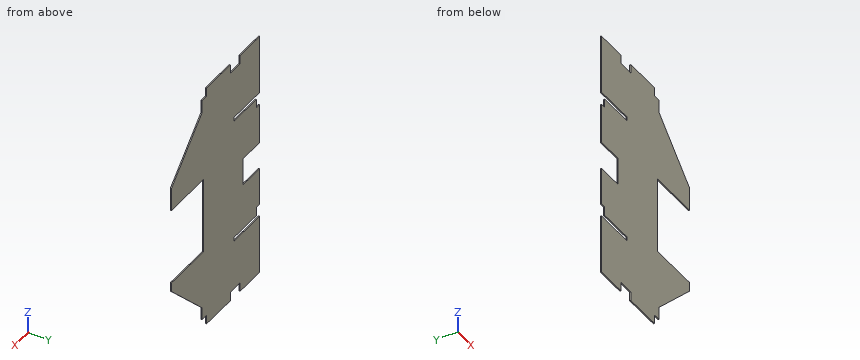
Autodesk Inventor part; units mm, degrees
ref_plane "YZ Plane" through (0, 0, 0) normal (1, 0, 0) x (0, 1, 0)
ref_plane "XZ Plane" through (0, 0, 0) normal (0, 1, 0) x (-1, 0, 0)
ref_plane "XY Plane" through (0, 0, 0) normal (0, 0, 1) x (1, 0, 0)
sketch "Sketch1" plane through (0, 0, 0) normal (0, 1, 0) x (-1, 0, 0)
  line L0 (234.95, 355.6) -> (-234.95, 355.6)
  line L1 (-234.95, 355.6) -> (-234.95, -355.6)
  line L2 (-234.95, -355.6) -> (234.95, -355.6)
  line L3 (234.95, -355.6) -> (234.95, 355.6)
  line L4 (234.95, 355.6) -> (-234.95, -355.6) construction
  line L5 (-234.95, 355.6) -> (234.95, -355.6) construction
  point P0 (0, 0)
  dimension "d0" = 469.9
  dimension "d1" = 711.2
extrude "Plate1" add sketch "Sketch1" along normal blind 3.048
sketch "Sketch3" plane through (0, 3.048, 0) normal (0, 1, 0) x (1, 0, 0)
  line L0 (234.95, -355.6) -> (-234.95, -355.6)
  point P0 (0, 0)
sketch "Sketch4" plane through (0, 0, 0) normal (0, -1, 0) x (1, 0, 0)
  line L0 (-234.95, 355.6) -> (234.95, 355.6)
  line L1 (-234.95, -355.6) -> (-234.95, 355.6)
  line L2 (234.95, -355.6) -> (-234.95, -355.6)
  line L3 (234.95, 355.6) -> (234.95, -355.6)
  line L4 (-234.95, 355.6) -> (234.95, 355.6)
  line L5 (25.4, 355.6) -> (25.4, 294.64)
  line L6 (165.1, 101.6) -> (234.95, 101.6)
  line L7 (234.95, 355.6) -> (234.95, -355.6)
  line L8 (25.4, 294.64) -> (165.1, 154.94)
  line L9 (25.4, 294.64) -> (222.9656, 294.64) construction
  line L10 (165.1, 154.94) -> (165.1, 101.6)
  line L11 (234.95, 0) -> (-234.95, 0)
  line L12 (-234.95, -355.6) -> (-234.95, 355.6)
  line L13 (25.4, -355.6) -> (25.4, -294.64)
  line L14 (165.1, -127) -> (234.95, -127)
  line L15 (25.4, -294.64) -> (165.1, -154.94)
  line L16 (25.4, -294.64) -> (222.9656, -294.64) construction
  line L17 (165.1, -154.94) -> (165.1, -127)
  line L18 (-234.95, 184.15) -> (-120.65, 184.15)
  line L19 (-120.65, 184.15) -> (-120.65, 177.8)
  line L20 (-120.65, 177.8) -> (-222.25, 177.8)
  line L21 (-222.25, 177.8) -> (-222.25, 152.4)
  line L22 (-222.25, 152.4) -> (-234.95, 152.4)
  line L23 (-234.95, 149.86) -> (-219.71, 149.86)
  line L24 (-219.71, 149.86) -> (-219.71, 175.26)
  line L25 (-219.71, 175.26) -> (-118.11, 175.26)
  line L26 (-118.11, 175.26) -> (-118.11, 186.69)
  line L27 (-118.11, 186.69) -> (-234.95, 186.69)
  line L28 (165.1, -129.54) -> (20.32, -129.54)
  line L29 (20.32, -129.54) -> (20.32, 88.9)
  line L30 (20.32, 88.9) -> (165.1, 88.9)
  line L31 (165.1, 101.6) -> (165.1, 88.9)
  line L32 (-234.95, -184.15) -> (-120.65, -184.15)
  line L33 (-120.65, -184.15) -> (-120.65, -177.8)
  line L34 (-120.65, -177.8) -> (-222.25, -177.8)
  line L35 (-222.25, -177.8) -> (-222.25, -152.4)
  line L36 (-222.25, -152.4) -> (-234.95, -152.4)
  line L37 (-234.95, -149.86) -> (-219.71, -149.86)
  line L38 (-219.71, -149.86) -> (-219.71, -175.26)
  line L39 (-219.71, -175.26) -> (-118.11, -175.26)
  line L40 (-118.11, -175.26) -> (-118.11, -186.69)
  line L41 (-118.11, -186.69) -> (-234.95, -186.69)
  line L42 (-158.75, 35.56) -> (-158.75, -43.18)
  line L43 (-158.75, -43.18) -> (-234.95, -43.18)
  line L44 (-158.75, 35.56) -> (-234.95, 35.56)
  line L45 (25.4, 330.2) -> (6.35, 330.2)
  line L46 (6.35, 330.2) -> (6.35, 355.6)
  line L47 (25.4, -330.2) -> (6.35, -330.2)
  line L48 (6.35, -330.2) -> (6.35, -355.6)
  line L49 (234.95, -355.6) -> (-234.95, -355.6)
  point P0 (0, 0)
  dimension "d3" = 209.55
  dimension "d4" = 254
  dimension "d5" = 45
  dimension "d6" = 60.96
  dimension "d9" = 69.85
  dimension "d12" = 45
  dimension "d13" = 209.55
  dimension "d14" = 228.6
  dimension "d15" = 69.85
  dimension "d16" = 60.96
  dimension "d17" = 171.45
  dimension "d18" = 114.3
  dimension "d19" = 6.35
  dimension "d21" = 101.6
  dimension "d22" = 25.4
  dimension "d23" = 2.54
  dimension "d26" = 144.78
  dimension "d31" = 12.7
  dimension "d32" = 114.3
  dimension "d33" = 171.45
  dimension "d34" = 6.35
  dimension "d35" = 101.6
  dimension "d36" = 25.4
  dimension "d37" = 2.54
  dimension "d38" = 76.2
  dimension "d39" = 35.56
  dimension "d40" = 43.18
  dimension "d41" = 2.54
  dimension "d42" = 25.4
  dimension "d43" = 19.05
  dimension "d44" = 25.4
  dimension "d45" = 19.05
extrude "Cut1" cut sketch "Sketch4" against normal blind 3.048 contours L27 L26 L25 L24 L23 L1 L22 L21 L20 L19 L18 | L0 L3 L6 L10 L8 L5 | L18 L19 L20 L21 L22 L1 | L3 L11 L29 L30 L31 L6 | L3 L14 L17 L28 L29 L11 | L44 L42 L11 L1 | L3 L2 L13 L15 L17 L14 | L11 L42 L43 L1 | L37 L38 L39 L40 L41 L1 L32 L33 L34 L35 L36 | L36 L35 L34 L33 L32 L1
sketch "Sketch5" plane through (0, 0, 0) normal (0, -1, 0) x (1, 0, 0)
  line L0 (25.4, 355.6) -> (25.4, 294.64)
  line L1 (25.4, 294.64) -> (165.1, 154.94)
  line L2 (165.1, 154.94) -> (165.1, 88.9)
  line L3 (165.1, 88.9) -> (20.32, 88.9)
  line L4 (20.32, 88.9) -> (20.32, -129.54)
  line L5 (20.32, -129.54) -> (165.1, -129.54)
  line L6 (165.1, -129.54) -> (165.1, -154.94)
  line L7 (165.1, -154.94) -> (25.4, -294.64)
  line L8 (25.4, -294.64) -> (25.4, -355.6)
  line L9 (25.4, -355.6) -> (-234.95, -355.6)
  line L10 (-234.95, -355.6) -> (-234.95, -186.69)
  line L11 (-234.95, -186.69) -> (-118.11, -186.69)
  line L12 (-118.11, -186.69) -> (-118.11, -175.26)
  line L13 (-118.11, -175.26) -> (-219.71, -175.26)
  line L14 (-219.71, -175.26) -> (-219.71, -149.86)
  line L15 (-219.71, -149.86) -> (-234.95, -149.86)
  line L16 (-234.95, -149.86) -> (-234.95, -43.18)
  line L17 (-234.95, -43.18) -> (-158.75, -43.18)
  line L18 (-158.75, -43.18) -> (-158.75, 35.56)
  line L19 (-158.75, 35.56) -> (-234.95, 35.56)
  line L20 (-234.95, 35.56) -> (-234.95, 149.86)
  line L21 (-234.95, 149.86) -> (-219.71, 149.86)
  line L22 (-219.71, 149.86) -> (-219.71, 175.26)
  line L23 (-219.71, 175.26) -> (-118.11, 175.26)
  line L24 (-118.11, 175.26) -> (-118.11, 186.69)
  line L25 (-118.11, 186.69) -> (-234.95, 186.69)
  line L26 (-234.95, 186.69) -> (-234.95, 355.6)
  line L27 (-234.95, 355.6) -> (25.4, 355.6)
  line L28 (25.4, -355.6) -> (-234.95, -355.6)
  line L29 (25.4, -355.6) -> (6.35, -355.6)
  line L30 (6.35, -355.6) -> (6.35, -330.2)
  line L31 (6.35, -330.2) -> (25.4, -330.2)
  line L32 (25.4, -330.2) -> (25.4, -355.6)
  line L33 (-234.95, 355.6) -> (25.4, 355.6)
  line L34 (25.4, 355.6) -> (6.35, 355.6)
  line L35 (6.35, 355.6) -> (6.35, 330.2)
  line L36 (6.35, 330.2) -> (25.4, 330.2)
  line L37 (25.4, 330.2) -> (25.4, 355.6)
  line L38 (-146.05, -355.6) -> (-101.6, -355.6)
  line L39 (-101.6, -355.6) -> (-101.6, -330.2)
  line L40 (-101.6, -330.2) -> (-146.05, -330.2)
  line L41 (-146.05, -330.2) -> (-146.05, -355.6)
  line L42 (-146.05, 355.6) -> (-101.6, 355.6)
  line L43 (-101.6, 355.6) -> (-101.6, 330.2)
  line L44 (-101.6, 330.2) -> (-146.05, 330.2)
  line L45 (-146.05, 330.2) -> (-146.05, 355.6)
  point P0 (0, 0)
  dimension "d46" = 19.05
  dimension "d47" = 25.4
  dimension "d48" = 19.05
  dimension "d49" = 25.4
  dimension "d52" = 44.45
  dimension "d53" = 25.4
  dimension "d54" = 88.9
  dimension "d55" = 44.45
  dimension "d56" = 25.4
  dimension "d57" = 88.9
extrude "Cut2" cut sketch "Sketch5" against normal blind 3.048 contours L0 L36 L35 L27 | L43 L44 L45 L27 | L8 L9 L30 L31 | L9 L41 L40 L39
equation "\"d10\" = Thickness"
equation "\"d2\" = Thickness"
equation "\"BendRadius\" = Thickness"
equation "\"BendReliefWidth\" = Thickness"
equation "\"BendReliefDepth\" = 0.5 * Thickness"
equation "\"CornerReliefSize\" = 4 * Thickness"
equation "\"MinimumRemnant\" = 2 * Thickness"
equation "\"TransitionRadius\" = BendRadius"
equation "\"JacobiRadiusSize\" = BendRadius"
equation "\"GapSize\" = Thickness"
properties part number "DB1-015" material "Polycarbonate, Smoke"
Model file for the job. Use its own axes, mm. Coordinates: 2 decimals unless noted, no trailing zeros. Loops run counter-clockwise (first coordinate to the right, second up) from the corner with the lowest first, then second, coordinate; pieces in that order, holes last. Notation, with made-up numbers: (-23, 36) -> (31, 36) arc R17 ccw to (31, 61) -> close; hole circle Ø6 at (-34, 86.5). An arc over 180 degrees is marked (long way). Answer as a JSON object with one key per item and string values.
Q1. Cut at B-B (x = -136.5). List the corners of the cut face in (y, z).
Report:
{"outline": "(0, -330.2) -> (3.05, -330.2) -> (3.05, -186.69) -> (0, -186.69) -> close; (0, -175.26) -> (3.05, -175.26) -> (3.05, 175.26) -> (0, 175.26) -> close; (0, 186.69) -> (3.05, 186.69) -> (3.05, 330.2) -> (0, 330.2) -> close"}
Q2. Flat gauge pins, fed straight in: P1, Ø0.9, axis at y = 2, z = -345, coming from the +X side; P2, Ø1.5, axis at y = 2.5, z = 165, coming from the -X side; P3, Ø0.9, axis at x = -133, y = 1, coming from the -Z side. Where does each tip first touch, or does it go through?
Report:
{"P1": "stops at x = 6.35", "P2": "stops at x = -219.71", "P3": "stops at z = -330.2"}
Q3. Probe probe 1 along Z at (x, y) = (-199, 0.8); probe 2 along Z at (x, y) = (-140, 2.65); probe 3 along X at (y, z) = (0.95, -16.5). List the from-to ranges inside material, lowest first.
Report:
{"probe 1": "z = -355.6 to -186.69, -175.26 to -43.18, 35.56 to 175.26, 186.69 to 355.6", "probe 2": "z = -330.2 to -186.69, -175.26 to 175.26, 186.69 to 330.2", "probe 3": "x = -158.75 to 20.32"}
Q4. Cut at C-C (x = -189). List the corners of the cut face in (y, z).
Report:
{"outline": "(0, -355.6) -> (3.05, -355.6) -> (3.05, -186.69) -> (0, -186.69) -> close; (0, -175.26) -> (3.05, -175.26) -> (3.05, -43.18) -> (0, -43.18) -> close; (0, 35.56) -> (3.05, 35.56) -> (3.05, 175.26) -> (0, 175.26) -> close; (0, 186.69) -> (3.05, 186.69) -> (3.05, 355.6) -> (0, 355.6) -> close"}
Q5. Cut at A-A (x = 72). List the corners of the cut face in (y, z), and give its area (3 significant figures).
Report:
{"outline": "(0, -248.04) -> (3.05, -248.04) -> (3.05, -129.54) -> (0, -129.54) -> close; (0, 88.9) -> (3.05, 88.9) -> (3.05, 248.04) -> (0, 248.04) -> close", "area": "846 mm2"}
Q6. Cut at D-D (z = -62.5). List the corners of the cut face in (x, y), and give its area (3 significant figures).
Report:
{"outline": "(-234.95, 0) -> (20.32, 0) -> (20.32, 3.05) -> (-234.95, 3.05) -> close", "area": "778 mm2"}
